from build123d import *

# Parameters (mm, degrees)
F3_D            = 12.7
F3_COPIES_COUNT = 10


# Not quite as in the source:
# - a pattern or mirror of a feature is missing from the dataset's text; its kind, count and spacing are read off the source's solid


with BuildPart() as f1:
    # F0 (on Front) → F1 (revolve)
    with BuildSketch(Plane.XZ):
        Polygon((-25.4, 0), (0, 0), (0, 50.172699946), (-12.7, 50.172699946), (-12.7, 12.072699946), (-25.4, 12.072699946), align=None)
    revolve(axis=Axis((-12.7, 0, -13.327300054), (-1, 0, 0)))

    # F3 (through all)
    with Locations(Plane.YZ):
        with Locations((0, 28.582699946)):
            f3 = Hole(F3_D / 2)

    # F3_copies: F3 ×10 about axis
    f3_copies_axis = Axis((0, 0, -13.3273), (1, 0, 0))
    for i in range(1, F3_COPIES_COUNT):
        add(f3.rotate(f3_copies_axis, i * 360 / F3_COPIES_COUNT), mode=Mode.SUBTRACT)


solid = f1.part
The model under review builds one solid part; all positions refer to its coordinate system, in mm. A direction names the side the tool comes from. Coordinates: 2 decimals unless noted, no trailing zeros. Write each loop counter-clockwise with the first axis right and the second up, starting at its lowest first coordinate (ties: lowest second). Pieces come first, ordered by that corner, then holes. Notation, with made-up numbers: (48, -38.5) -> (53, -38.5) arc R16 cw to (53, -32.5) -> close; hole circle Ø8 at (-29.75, 88). An arc over 180 degrees is marked (long way). Answer in a Markdown table with one row per item.
1. Draft analysis for pull direction Z (two halves, no side actions). For faces 3 (the cylindrical face through (-6.44, -24.32, 45.33)), 4 (the flat face through (0, 15, -12)), 5 (the cylindrical face through (-6.439, 1.377, 22.384)), state which applies: +Z half, -Z half, draft (parallel to the pull), parting line (faces both ways), or undercut.
Answers below:
| item | result |
|---|---|
| face 3 | parting line |
| face 4 | draft |
| face 5 | undercut |
2. Wall thickness on probe 1 along Z at (x, y) = (-3, 28.5); probe 2 along Y at (x, z) = (-10.5, 25); probe 3 along Y at (x, z) = (-22.5, -13): over which ranges is each line inside the solid? List them lowest first. Write a range as [from, to].
Answers below:
| item | result |
|---|---|
| probe 1 | z = [-70.07, -52.27], [-42.2, 15.54], [25.62, 43.42] |
| probe 2 | y = [-50.63, -29.19], [-20.08, -5.24], [5.24, 20.08], [29.19, 50.63] |
| probe 3 | y = [-25.4, -13.32], [13.32, 25.4] |
3. We need section B-B, the plane x = -9. Give the number of separate pieces and of enclosed holes in the cut face, and give its area (3 significant figures).
Answers below:
| item | result |
|---|---|
| separate pieces | 1 |
| enclosed holes | 11 |
| area | 10,800 mm^2 |
4. We need section C-C, the plane x = -19.5. State the section outline as (y, z) points, and give its area (3 significant figures).
Answers below:
| item | result |
|---|---|
| outline | circle Ø50.8 at (0, -13.33); hole circle Ø26.65 at (0, -13.33) |
| area | 1,470 mm^2 |
5. We need section D-D, the plane z = 9.5. State the section outline as (x, y) points.
Answers below:
| item | result |
|---|---|
| outline | (-25.4, -11.14) -> (-12.7, -11.14) -> (-12.7, -59.26) -> (0, -59.26) -> (0, 59.26) -> (-12.7, 59.26) -> (-12.7, 11.14) -> (-25.4, 11.14) -> close |
6. Clearance check with flat-ended pins moving along their axes: pin 1 Ø16.5 at (y, z) = (39.86, -0.38) entering from -X; pin 2 Ø3 at (x, y) = (-3, 50) entering from -Z; pin 3 Ø8 at (x, z) = (-13.5, -51.5) entering from -Y; pin 4 Ø4 at (y, z) = (24.5, 27.5) entering from +X. State where each tip first meets the part, or that it passes through.
Answers below:
| item | result |
|---|---|
| pin 1 | stops at x = -12.7 |
| pin 2 | stops at z = -54.32 |
| pin 3 | stops at y = -53.47 |
| pin 4 | stops at x = 0 |
7. For faces 1 (the flat face through (-25.4, -11, -2)), 2 (the flat face through (-12.7, 1, 14)), list the 3-axis set-ups (+Z, -Z, +X, -X, +Y, -Y) from which the entire face can be reached by the end or side of a thin tool; tool diameter is ignored.
Answers below:
| item | result |
|---|---|
| face 1 | +Z, -Z, -X, +Y, -Y |
| face 2 | -X |
8. We need section A-A, the plane y = 0. State the section outline as (x, z) points, and give its area (3 significant figures).
Answers below:
| item | result |
|---|---|
| outline | (-25.4, -38.73) -> (-12.7, -38.73) -> (-12.7, -48.89) -> (0, -48.89) -> (0, -26.65) -> (-25.4, -26.65) -> close; (-25.4, 0) -> (0, 0) -> (0, 22.23) -> (-12.7, 22.23) -> (-12.7, 12.07) -> (-25.4, 12.07) -> close; (-12.7, -76.83) -> (0, -76.83) -> (0, -61.59) -> (-12.7, -61.59) -> close; (-12.7, 34.93) -> (0, 34.93) -> (0, 50.17) -> (-12.7, 50.17) -> close |
| area | 1,260 mm^2 |
